Source: CAD feature listing. Evaluate the final solid. Frame: model axes, mm. A direction names the side the tool comes from. Coordinates: 2 decimals unless noted, no trailing zeros. Write each loop counter-clockwise with the first axis right and the second up, starting at its lowest first coordinate (ties: lowest second). Pieces come first, ordered by that corner, then holes. Notation, with made-up numbers: M 59,-7.5 L 67,-7.5 A38 cw 67,31.5 Z; hole C 60,11 d9. An arc over 180 degrees is marked long. Answer as CSV lines item,"result". Start each with the question number.
1. Mould query, pull axis X, two halves, no side actions, for faces 5 (the face through (43.85, -2.28, 12.88)), 6 (the face through (-13, 19.236, 63)), 7 (the face through (-6.551, 26, 63)), 8 (the face through (13.521, 27, 63)). Classes: pulls with the +X half, pulls with the -X half, needs draft (parallel to the pull), parting line crosses it, or undercut.
2. Contact query for flat-ended pins moving along their axis: pin 1 Ø10 at (y, z) = (-3.5, 103) entering from +X; pin 2 Ø1.5 at (y, z) = (-25.5, 44) entering from +X; pin 3 Ø8 at (y, z) = (-15, 33) entering from -X; pin 4 Ø15 at (x, z) = (21, 65) entering from -Y. Output: stop coordinate, or through.
3. Section A-A on z = 89. Return the cut outline in (x, y), plus the area to 3 significant figures.
4. Reachability of faces 1 (the face through (-18.26, -27, 63)), 2 (the face through (27.181, 27, 63)), 3 (the face through (-4.321, -27, 63)), 4 (the face through (-7, 33.454, 87)) from +Z, -Z, +X, -X, +Y, -Y: full face, straight path, thin tool, end or side. Return the list, or none.
5. Line query: probe 1 along Z at (x, y) = (-3, -25); probe 2 along Y at (x, z) = (-18, 90.5); probe 3 along Z at (x, y) = (21.5, -36.5). Output: solid intervals per line, ascending. Write a range as [from, to].
```python
from build123d import *

# Parameters (mm, degrees)
F0_W     = 104.2639054358
F0_H     = 126.0087862611
F1_DEPTH = 25.4
F2_SIZE  = 25.39999
F3_W     = 12.2663415968
F3_H     = 14.2178032547
F3_W_2   = 13.6602446437
F3_H_2   = 11.9875594974
F3_W_3   = 13.9390230179
F3_H_3   = 12.8239002079
F3_W_4   = 11.9875576347
F3_H_4   = 11.9875632226
F4_DEPTH = 76.2
F5_W     = 44.9166167527
F5_H     = 65.0939904153
F6_DEPTH = 25.4


# Not quite as in the source:
# - a fillet or chamfer is up to 0.001 mm smaller than in the source, because OpenCascade refuses the exact size


with BuildPart() as f1:
    # F0 (on Top) → F1 (new body)
    with BuildSketch(Plane.XY):
        with Locations((4.5998785645, -1.3939030468)):
            Rectangle(F0_W, F0_H)
    extrude(amount=F1_DEPTH)

    # F2 (size 25.4 in the source; OpenCascade refuses exactly that, so slightly less here)
    f2_edges = [f1.edges().sort_by_distance(p)[0] for p in [
        (-47.532074, -1.393903, 25.4),
        (4.599879, -64.398296, 25.4),
        (56.731831, -1.393903, 25.4),
        (4.599879, 61.61049, 25.4),
    ]]
    chamfer(f2_edges, length=F2_SIZE)

    # F3 (on face) → F4 (join)
    with BuildSketch(Plane.XY.offset(25.4)):
        with Locations((-12.6845128834, 26.3447565958)):
            Rectangle(F3_W, F3_H)
        with Locations((20.3509759158, 26.6235359013)):
            Rectangle(F3_W_2, F3_H_2)
        with Locations((-11.2906098366, -26.7629260197)):
            Rectangle(F3_W_3, F3_H_3)
        with Locations((20.3509749845, -25.7871951908)):
            Rectangle(F3_W_4, F3_H_4)
    extrude(amount=F4_DEPTH)

    # F5 (on face) → F6 (join)
    with BuildSketch(Plane.XY.offset(101.6)):
        with Locations((3.6406246945, 0.9066630155)):
            Rectangle(F5_W, F5_H)
    extrude(amount=F6_DEPTH)


solid = f1.part
```
Values:
1,face 5,"pulls with the +X half"
1,face 6,"needs draft"
1,face 7,"undercut"
1,face 8,"undercut"
2,pin 1,"x = 26.1"
2,pin 2,"x = 26.34"
2,pin 3,"through"
2,pin 4,"y = -31.78"
3,outline,"M -18.82,19.24 L -6.55,19.24 L -6.55,33.45 L -18.82,33.45 Z; M -18.26,-33.17 L -4.32,-33.17 L -4.32,-20.35 L -18.26,-20.35 Z; M 13.52,20.63 L 27.18,20.63 L 27.18,32.62 L 13.52,32.62 Z; M 14.36,-31.78 L 26.34,-31.78 L 26.34,-19.79 L 14.36,-19.79 Z"
3,area,"661 mm²"
4,face 1,"-X, -Y"
4,face 2,"+Z, +X, +Y, -Y"
4,face 3,"+Y, -Y"
4,face 4,"+Z, +X, -X, +Y"
5,probe 1,"[0, 25.4], [101.6, 127]"
5,probe 2,"[-33.17, -20.35], [19.24, 33.45]"
5,probe 3,"[0, 25.4]"
